Geometry check sheet. Reference: the model listing, model coordinates, mm. Round coordinates to 2 decimals unless told otherwise and drop trailing zeros. Order: outer loops, then holes, each group sorted by start corner. A loop starts at its lowest first (then second) coordinate and runs counter-clockwise, first axis right, second up.
Autodesk Inventor part; units mm, degrees
ref_plane "YZ Plane" through (0, 0, 0) normal (1, 0, 0) x (0, 1, 0)
ref_plane "XZ Plane" through (0, 0, 0) normal (0, 1, 0) x (-1, 0, 0)
ref_plane "XY Plane" through (0, 0, 0) normal (0, 0, 1) x (1, 0, 0)
sketch "Absorber-Base" plane through (0, 0, 0) normal (0, 0, 1) x (1, 0, 0)
  line L0 (-9.2424, 9.2424) -> (9.2424, 9.2424)
  line L1 (9.2424, 9.2424) -> (9.2424, -9.2424)
  line L2 (9.2424, -9.2424) -> (-9.2424, -9.2424)
  line L3 (-9.2424, -9.2424) -> (-9.2424, 9.2424)
  line L4 (-9.2424, 9.2424) -> (9.2424, -9.2424) construction
  line L5 (9.2424, 9.2424) -> (-9.2424, -9.2424) construction
  point P0 (0, 0)
  dimension "d0" = 18.4849
extrude "Gesamtvolumen" add sketch "Absorber-Base" along normal blind 23
sketch "Skizze2" plane through (0, 0, 0) normal (0, 1, 0) x (-1, 0, 0)
  line L0 (-28, 0) -> (28, 0)
  line L1 (9.2424, 0) -> (9.2424, 23)
  line L2 (-9.2424, 0) -> (-9.2424, 23)
  line L3 (9.2424, 0) -> (-9.2424, 0)
  line L4 (-9.2424, 0) -> (-9.2424, 5)
  line L5 (-9.2424, 5) -> (9.2424, 5)
  line L6 (9.2424, 5) -> (9.2424, 0)
  line L7 (-9.2424, 23) -> (9.2424, 23)
  line L8 (0, 23) -> (9.2424, 5)
  line L9 (0, 23) -> (-9.2424, 5)
  point P0 (0, 0)
  point P1 (9.2424, 5)
  dimension "d6" = 5
extrude "Cutaway" cut sketch "Skizze2" along normal mid plane 18.4848 contours L2 L7 L9 | L8 L7 L1
pattern_circular "Runde Anordnung1" count 2 over 90 about axis through (0, 0, -10) along (0, 0, 1) of "Cutaway"
equation "\"d0\" = Base_Seitenlänge"
equation "\"d1\" = Gesamthöhe"
equation "\"d6\" = Base_Höhe"
equation "\"d7\" = Base_Seitenlänge"
equation "\"Base_Seitenlänge\" = 18.48485"
equation "\"Base_Höhe\" = 5"
equation "\"Gesamthöhe\" = 23"
properties part number "Absorber - SEA-PM3"
(1) Material ranges on line 1 (Y direction, x = 3.5, z = 9); line 2 (Z direction, x = 1.25, y = 0); line 3 (Z direction, x = -3.5, y = -2.25), recorded low to high.
Returned:
line 1: y = -7.19 to 7.19
line 2: z = 0 to 20.57
line 3: z = 0 to 16.18
(2) Sectioned sample at C-C, the plane z = 16.25. Record the cut outline in (x, y).
Returned:
outline: (-3.47, -3.47) - (3.47, -3.47) - (3.47, 3.47) - (-3.47, 3.47) - close
(3) Depth check by flat-ended pin: P1, Ø2, axis at x = -6, z = 11.5, coming from the -Y side; P2, Ø6, axis at y = -2, z = 19, coming from the +X side; P3, Ø6, axis at x = -1.5, z = 10.5, coming from the -Y side. Enter the tip coordinate at first touch or a pass-through.
Returned:
P1: stops at y = -6.42
P2: stops at x = 3.59
P3: stops at y = -7.96
(4) Sectioned sample at A-A, the plane x = -5.5. Record the cut outline in (y, z).
Returned:
outline: (-9.24, 0) - (9.24, 0) - (9.24, 5) - (5.5, 12.29) - (-5.5, 12.29) - (-9.24, 5) - close
(5) Sectioned sample at B-B, the plane y = 2.5. Record the cut outline in (x, z), and give its area (3 significant figures).
Returned:
outline: (-9.24, 0) - (9.24, 0) - (9.24, 5) - (2.5, 18.13) - (-2.5, 18.13) - (-9.24, 5) - close
area: 247 mm2
(6) Sectioned sample at D-D, the plane z = 21.75. Record the cut outline in (x, y), and give its area (3 significant figures).
Returned:
outline: (-0.64, -0.64) - (0.64, -0.64) - (0.64, 0.64) - (-0.64, 0.64) - close
area: 1.65 mm2
